For this review, take the finished solid that the model builds, in its own axes (mm). Face numbers are marked on the shaded views. Give positions to 0.01 mm unless a question says otherwise; leave off trailing zeros. Order: outer loops, then holes, each group sorted by start corner. A loop starts at its lowest first (then second) coordinate and runs counter-clockwise, first axis right, second up. Notation, with made-up numbers: (1.25, 5) - (5.25, 5) arc R14 cw to (5.25, 25) - close; hole circle Ø11 at (-17, 89). An arc over 180 degrees is marked (long way). One line per item, written item: value.
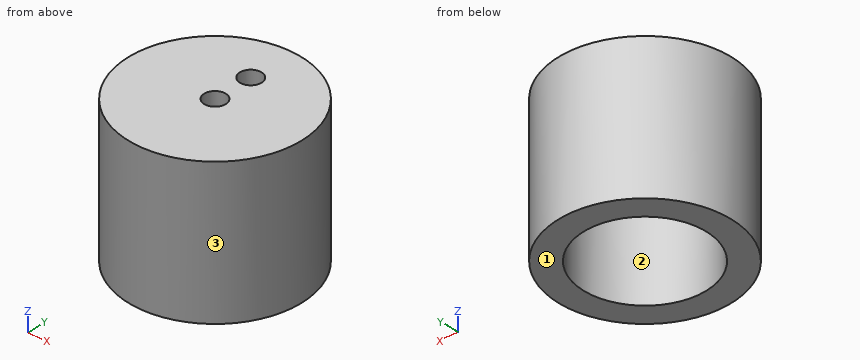
```python
from build123d import *

# Parameters (mm, degrees)
F0_R     = 6
F0_R_2   = 4.25
F1_DEPTH = 10
F2_DEPTH = 8
F3_D     = 1.5


with BuildPart() as f1:
    # F0 (on Top) → F1 (new body)
    with BuildSketch(Plane.XY):
        with Locations((0, -0.5465864819)):
            Circle(F0_R)
        with Locations((0, -0.5465864819)):
            Circle(F0_R_2, mode=Mode.SUBTRACT)
        with Locations((0, -0.5465864819)):
            Circle(F0_R_2)
    extrude(amount=F1_DEPTH)

    # F0 (on Top) → F2 (cut)
    with BuildSketch(Plane.XY):
        with Locations((0, -0.5465864819)):
            Circle(F0_R_2)
    extrude(amount=F2_DEPTH, mode=Mode.SUBTRACT)

    # F3 (through all)
    with Locations(Plane(origin=(0, 0, 0), x_dir=(1, 0, 0), z_dir=(0, 0, -1))):
        with Locations((0, 0.5465864819), (0, -2.2034135181)):
            Hole(F3_D / 2)


solid = f1.part
```
(1) Take a section at B-B (y = 1.25). Write out the cut boundary in (x, z).
Answers below:
outline: (-5.72, 0) - (-3.85, 0) - (-3.85, 8) - (3.85, 8) - (3.85, 0) - (5.72, 0) - (5.72, 10) - (-5.72, 10) - close
(2) For P1, Ø5, axis at y = 4, z = 6, coming from the +X side; P2, Ø2, axis at x = -3.5, z = 3, coming from the -Y side; P3, Ø6, axis at y = 2, z = 4.5, coming from the -X side; P4, Ø1, axis at x = 2.5, z = 2, coming from the +Y side, all flat-tipped, find the tip position at first contact; note any pin that passes through.
Answers below:
P1: stops at x = 5.64
P2: stops at y = -6
P3: stops at x = -6
P4: stops at y = 5.11
(3) Draft analysis for pull direction X (two halves, no side actions). For the marked faces 1, 2 and 3, state which applies: pulls with the +X half, pulls with the -X half, needs draft (parallel to the pull), parting line crosses it, or undercut.
Answers below:
face 1: needs draft
face 2: undercut
face 3: parting line crosses it
(4) Take a section at D-D (z = 2.75). Write out the cut boundary in (x, y).
Answers below:
outline: circle Ø12 at (0, -0.55); hole circle Ø8.5 at (0, -0.55)
(5) Take a section at A-A (x = 0). Write out the cut boundary in (y, z), then the cut area to 3 significant figures.
Answers below:
outline: (-6.55, 0) - (-4.8, 0) - (-4.8, 8) - (-1.3, 8) - (-1.3, 10) - (-6.55, 10) - close; (0.2, 8) - (1.45, 8) - (1.45, 10) - (0.2, 10) - close; (2.95, 8) - (3.7, 8) - (3.7, 0) - (5.45, 0) - (5.45, 10) - (2.95, 10) - close
area: 46.0 mm^2
(6) Wall thickness on line 1 (Y direction, x = 0, z = 8.5); line 2 (Y direction, x = 0.25, z = 9); line 3 (Z direction, x = 2.25, y = -0.5): over which ranges is each line inside the solid? List them lowest first. Write a range as from..to.
Answers below:
line 1: y = -6.55..-1.3, 0.2..1.45, 2.95..5.45
line 2: y = -6.54..-1.25, 0.16..1.5, 2.91..5.45
line 3: z = 8..10
(7) Take a section at C-C (x = 2.5). Write out the cut boundary in (y, z), then the cut area to 3 significant figures.
Answers below:
outline: (-6, 0) - (-3.98, 0) - (-3.98, 8) - (2.89, 8) - (2.89, 0) - (4.91, 0) - (4.91, 10) - (-6, 10) - close
area: 54.1 mm^2
